Model file for the job. Use its own axes, mm. Coordinates: 2 decimals unless noted, no trailing zeros. Order: outer loops, then holes, each group sorted by start corner. A loop starts at its lowest first (then second) coordinate and runs counter-clockwise, first axis right, second up. Notation, with made-up numbers: (-11.5, 16) - (-3.5, 16) arc R5 cw to (-3.5, 24) - close; hole circle Ø7 at (-32, -27). An arc over 180 degrees is marked (long way). Put each result on its own line as item: value. Start each with the question number.
```python
from build123d import *

# Parameters (mm, degrees)
F4_DEPTH = 2


# Not quite as in the source:
# - a feature of the source that left no trace in its solid (it failed there, or was rolled back) is left out


with BuildPart() as f2:
    # F1 (on Front) → F2 (revolve)
    with BuildSketch(Plane.XZ):
        with BuildLine():
            Line((0, 67), (0, 65))
            Line((0, 65), (15, 65))
            Line((15, 65), (15, 66))
            ThreePointArc((15, 66), (14.7071067812, 66.7071067812), (14, 67))
            Line((14, 67), (0, 67))
        make_face()
        with BuildLine():
            Line((0, 65), (0, 0))
            Line((0, 0), (18.2, 0))
            ThreePointArc((18.2, 0), (18.2707106781, 0.0292893219), (18.3, 0.1))
            Line((18.3, 0.1), (18.3, 59))
            ThreePointArc((18.3, 59), (17.9754446797, 61), (18.3, 63))
            Line((18.3, 63), (18.3, 64))
            ThreePointArc((18.3, 64), (18.0071067812, 64.7071067812), (17.3, 65))
            Line((17.3, 65), (15, 65))
            Line((15, 65), (0, 65))
        make_face()
    revolve(axis=Axis((0, 0, 33.5), (0, 0, 1)))

    # F3 (on face) → F4 (cut)
    with BuildSketch(Plane.XY.offset(67)):
        with BuildLine():
            ThreePointArc((-6.1588027163, 7.8783976227), (-6.8349323024, 9.3151975073), (-8.240042652, 10.0549339676))
            ThreePointArc((-8.240042652, 10.0549339676), (-11.2583302492, 6.5), (-12.8278495753, 2.1086192811))
            ThreePointArc((-12.8278495753, 2.1086192811), (-11.4846638338, 1.2616262534), (-9.9022938405, 1.3944807979))
            ThreePointArc((-9.9022938405, 1.3944807979), (-8.6602540378, 5), (-6.1588027163, 7.8783976227))
        make_face()
        with BuildLine():
            ThreePointArc((-3.7434911242, 9.2728784206), (0, 10), (3.7434911242, 9.2728784206))
            ThreePointArc((3.7434911242, 9.2728784206), (4.6497315314, 10.5768237606), (4.5878069233, 12.1635532487))
            ThreePointArc((4.5878069233, 12.1635532487), (0, 13), (-4.5878069233, 12.1635532487))
            ThreePointArc((-4.5878069233, 12.1635532487), (-4.6497315314, 10.5768237606), (-3.7434911242, 9.2728784206))
        make_face()
        with BuildLine():
            ThreePointArc((-9.9022938405, -1.3944807979), (-11.4846638338, -1.2616262534), (-12.8278495753, -2.1086192811))
            ThreePointArc((-12.8278495753, -2.1086192811), (-11.2583302492, -6.5), (-8.240042652, -10.0549339676))
            ThreePointArc((-8.240042652, -10.0549339676), (-6.8349323024, -9.3151975073), (-6.1588027163, -7.8783976227))
            ThreePointArc((-6.1588027163, -7.8783976227), (-8.6602540378, -5), (-9.9022938405, -1.3944807979))
        make_face()
        with BuildLine():
            ThreePointArc((-3.7434911242, -9.2728784206), (-4.6497315314, -10.5768237606), (-4.5878069233, -12.1635532487))
            ThreePointArc((-4.5878069233, -12.1635532487), (0, -13), (4.5878069233, -12.1635532487))
            ThreePointArc((4.5878069233, -12.1635532487), (4.6497315314, -10.5768237606), (3.7434911242, -9.2728784206))
            ThreePointArc((3.7434911242, -9.2728784206), (0, -10), (-3.7434911242, -9.2728784206))
        make_face()
        with BuildLine():
            ThreePointArc((6.1588027163, -7.8783976227), (6.8349323024, -9.3151975073), (8.240042652, -10.0549339676))
            ThreePointArc((8.240042652, -10.0549339676), (11.2583302492, -6.5), (12.8278495753, -2.1086192811))
            ThreePointArc((12.8278495753, -2.1086192811), (11.4846638338, -1.2616262534), (9.9022938405, -1.3944807979))
            ThreePointArc((9.9022938405, -1.3944807979), (8.6602540378, -5), (6.1588027163, -7.8783976227))
        make_face()
        with BuildLine():
            ThreePointArc((9.9022938405, 1.3944807979), (11.4846638338, 1.2616262534), (12.8278495753, 2.1086192811))
            ThreePointArc((12.8278495753, 2.1086192811), (11.2583302492, 6.5), (8.240042652, 10.0549339676))
            ThreePointArc((8.240042652, 10.0549339676), (6.8349323024, 9.3151975073), (6.1588027163, 7.8783976227))
            ThreePointArc((6.1588027163, 7.8783976227), (8.6602540378, 5), (9.9022938405, 1.3944807979))
        make_face()
    extrude(amount=-F4_DEPTH, mode=Mode.SUBTRACT)


solid = f2.part
```
Item 1: Wall check: line 1 along Z through (x, y) = (16, -2.5); line 2 along Y through (x, z) = (-2, 53); line 3 along Y through (x, z) = (-13, 47). Give the ranges that are in metal, low to high.
Item 2: Pull direction Y, two halves, no side cores. Call faces 1 (the face through (-13, 8, 65)), 2 (the face through (9, 6, 65)): pulls with the +Y half, pulls with the -Y half, needs draft (parallel to the pull), parting line crosses it, or undercut.
Item 3: Flat gauge pins, fed straight in: pin 1 Ø8 at (y, z) = (6, 10) entering from -X; pin 2 Ø5 at (y, z) = (-6.5, 13) entering from -X; pin 3 Ø2 at (x, z) = (14.5, 20.5) entering from -Y. Where does each tip first touch, or does it go through?
Item 4: Slice it at A-A, the plane z = 57. Give the cut face in (x, y).
Here are the results:
1. line 1: z = 0 to 65
1. line 2: y = -18.19 to 18.19
1. line 3: y = -12.88 to 12.88
2. face 1: needs draft
2. face 2: undercut
3. pin 1: stops at x = -18.19
3. pin 2: stops at x = -17.86
3. pin 3: stops at y = -12.35
4. outline: circle Ø36.6 at (0, 0)
